Work out the finished part from the listing and answer in its coordinate system (mm). Round coordinates to 2 decimals unless told otherwise and drop trailing zeros. Order: outer loops, then holes, each group sorted by start corner. A loop starts at its lowest first (then second) coordinate and runs counter-clockwise, first axis right, second up. Notation, with made-up numbers: (3, 10.25) - (10, 10.25) arc R14 ccw to (10, 19.25) - close; hole circle Ø11 at (30.25, 56.5). An arc over 180 degrees is marked (long way). Put each result on its own line as item: value.
```python
from build123d import *

# Parameters (mm, degrees)
SKETCH1_W           = 108.016753786
SKETCH1_H           = 50
SKETCH1_R           = 11
SKETCH1_R_2         = 1.75
BOSS_EXTRUDE1_DEPTH = 10
FILLET1_R           = 15


with BuildPart() as part:
    # Sketch1 → Boss-Extrude1 (new body)
    with BuildSketch(Plane(origin=(0, 0, 0), x_dir=(1, 0, 0), z_dir=(0, 1, 0))):
        with Locations((-25.991623107, 0)):
            Rectangle(SKETCH1_W, SKETCH1_H)
        Circle(SKETCH1_R, mode=Mode.SUBTRACT)
        with Locations((15.5, 15.5)):
            Circle(SKETCH1_R_2, mode=Mode.SUBTRACT)
        with Locations((-15.5, 15.5)):
            Circle(SKETCH1_R_2, mode=Mode.SUBTRACT)
        with Locations((-15.5, -15.5)):
            Circle(SKETCH1_R_2, mode=Mode.SUBTRACT)
        with Locations((15.5, -15.5)):
            Circle(SKETCH1_R_2, mode=Mode.SUBTRACT)
        with Locations((-65.5, 15.5)):
            Circle(SKETCH1_R_2, mode=Mode.SUBTRACT)
        with Locations((-34.5, 15.5)):
            Circle(SKETCH1_R_2, mode=Mode.SUBTRACT)
        with Locations((-34.5, -15.5)):
            Circle(SKETCH1_R_2, mode=Mode.SUBTRACT)
        with Locations((-65.5, -15.5)):
            Circle(SKETCH1_R_2, mode=Mode.SUBTRACT)
        with Locations((-50, 0)):
            Circle(SKETCH1_R, mode=Mode.SUBTRACT)
    extrude(amount=BOSS_EXTRUDE1_DEPTH)

    # Fillet1
    fillet1_edges = [part.edges().sort_by_distance(p)[0] for p in [
        (-80, 5, -25),
        (28.016753786, 5, -25),
        (28.016753786, 5, 25),
        (-80, 5, 25),
    ]]
    fillet(fillet1_edges, radius=FILLET1_R)


solid = part.part
```
1) A cutting plane is placed at D-D on x = -50. Write down the section's boundary in (y, z), then the cut area to 3 significant figures.
Findings below:
outline: (0, -25) - (10, -25) - (10, -11) - (0, -11) - close; (0, 11) - (10, 11) - (10, 25) - (0, 25) - close
area: 280 mm2
2) For a pull along X with two mould halves and no side action, classify faces 1 (the flat face through (28.017, 5, 0)), 2 (the cylindrical face through (-63.831, 4.93, -16.026)), 3 (the cylindrical face through (-75.72, 5.07, 20.49)) as pulls with the +X half, pulls with the -X half, needs draft (parallel to the pull), parting line crosses it, or undercut.
Findings below:
face 1: pulls with the +X half
face 2: undercut
face 3: pulls with the -X half
3) A cutting plane is placed at C-C on y = 8.5. Give the number of separate pieces and of enclosed holes in the cut face, then the cut area to 3 significant figures.
Findings below:
separate pieces: 1
enclosed holes: 10
area: 4,370 mm2
4) Given pin 1 Ø17.5 at (x, z) = (0, 0) entering from +Y; pin 2 Ø2 at (x, y) = (15, 4.5) entering from -Z, each flat-ended and moving along its own axis, determine where each tip first touches the part or whether it passes through.
Findings below:
pin 1: passes through
pin 2: stops at z = -24.97
5) Straight lines are drawn through the part: L1, parallel to Z at x = -34.5, y = 7; L2, parallel to X at y = 3.5, z = 0; L3, parallel to X at y = 4, z = 8.5. For each, find the intervals that lie inside material, in ascending order. Write a range as from..to.
Findings below:
L1: z = -25..-17.25, -13.75..13.75, 17.25..25
L2: x = -80..-61, -39..-11, 11..28.02
L3: x = -80..-56.98, -43.02..-6.98, 6.98..28.02
6) A cutting plane is placed at B-B on z = 0. Write down the section's boundary in (x, y).
Findings below:
outline: (-80, 0) - (-61, 0) - (-61, 10) - (-80, 10) - close; (-39, 0) - (-11, 0) - (-11, 10) - (-39, 10) - close; (11, 0) - (28.02, 0) - (28.02, 10) - (11, 10) - close
7) A cutting plane is placed at A-A on x = -15.5. Write down the section's boundary in (y, z).
Findings below:
outline: (0, -25) - (10, -25) - (10, -17.25) - (0, -17.25) - close; (0, -13.75) - (10, -13.75) - (10, 13.75) - (0, 13.75) - close; (0, 17.25) - (10, 17.25) - (10, 25) - (0, 25) - close
